Geometry: final body of the model. Coordinates: model frame, mm. A direction names the side the tool comes from. Give positions to 0.01 mm unless a question says otherwise; leave off trailing zeros. Order: outer loops, then holes, each group sorted by start corner. A loop starts at its lowest first (then second) coordinate and runs counter-clockwise, first axis right, second up. Notation, with made-up numbers: (60.5, 69) - (103.5, 69) arc R21 ccw to (103.5, 90) - close; hole circle Ø11 at (12.25, -26). An arc over 180 degrees is marked (long way). Use one line per item in the form item = value.
from build123d import *

# Parameters (mm, degrees)
F0_W      = 32
F0_H      = 9
F0_W_2    = 1
F1_DEPTH  = 6.5
F2_DEPTH  = 5.5
F3_DEPTH  = 4
F4_W      = 1
F4_H      = 1
F5_DEPTH  = 35
F6_DEPTH  = 33
F9_DEPTH  = 2
F4_W_2    = 9
F10_DEPTH = 33


with BuildPart() as f1:
    # F0 (on Top) → F1 (new body)
    with BuildSketch(Plane.XY):
        Polygon((4.2322745472, -4.5), (-27.7677254528, -4.5), (-28.7677254528, -4.5), (-28.7677254528, -6.5), (7.2322745472, -6.5), (7.2322745472, 6.5), (-28.7677254528, 6.5), (-28.7677254528, 4.5), (-27.7677254528, 4.5), (4.2322745472, 4.5), align=None)
        with Locations((-11.7677254528, 0)):
            Rectangle(F0_W, F0_H)
        with Locations((-28.2677254528, 0)):
            Rectangle(F0_W_2, F0_H)
    extrude(amount=F1_DEPTH)

    # F0 (on Top) → F2 (cut)
    with BuildSketch(Plane.XY):
        with Locations((-11.7677254528, 0)):
            Rectangle(F0_W, F0_H)
    extrude(amount=F2_DEPTH, mode=Mode.SUBTRACT)

    # F0 (on Top) → F3 (join)
    with BuildSketch(Plane.XY):
        Polygon((4.2322745472, -4.5), (-27.7677254528, -4.5), (-28.7677254528, -4.5), (-28.7677254528, -6.5), (7.2322745472, -6.5), (7.2322745472, 6.5), (-28.7677254528, 6.5), (-28.7677254528, 4.5), (-27.7677254528, 4.5), (4.2322745472, 4.5), align=None)
    extrude(amount=-F3_DEPTH)

    # F4 (on face) → F5 (cut)
    with BuildSketch(Plane(origin=(-28.7677254528, 0, 0), x_dir=(0, -1, 0), z_dir=(-1, 0, 0))):
        with Locations((-5, -1.5)):
            Rectangle(F4_W, F4_H)
    extrude(amount=-F5_DEPTH, mode=Mode.SUBTRACT)

    # F4 (on face) → F6 (cut)
    with BuildSketch(Plane(origin=(-28.7677254528, 0, 0), x_dir=(0, -1, 0), z_dir=(-1, 0, 0))):
        with Locations((-5, 1.5)):
            Rectangle(F4_W, F4_H)
        Polygon((-4.5, 1), (-4.5, 0), (0, 0), (0, 2), (-4.5, 2), align=None)
    extrude(amount=-F6_DEPTH, mode=Mode.SUBTRACT)

    # F7: F1 across plane


with BuildPart() as f1_1:
    add(f1.part)
    add(f1.part.mirror(Plane.XZ), mode=Mode.INTERSECT)

    # F8 (on face) → F9 (cut)
    with BuildSketch(Plane(origin=(4.2322745472, 0, 0), x_dir=(0, -1, 0), z_dir=(-1, 0, 0))):
        Polygon((4.5, 0), (-4.5, 0), (-4.5, -1), (-4.5, -2), (-4.5, -3), (4.5, -3), (4.5, -2), (4.5, -1), align=None)
    extrude(amount=-F9_DEPTH, mode=Mode.SUBTRACT)

    # F4 (on face) → F10 (join, through all)
    with BuildSketch(Plane(origin=(-28.7677254528, 0, 0), x_dir=(0, -1, 0), z_dir=(-1, 0, 0))):
        with Locations((0, -3.5)):
            Rectangle(F4_W_2, F4_H)
    extrude(amount=-F10_DEPTH)


solid = f1_1.part
(1) Pull-direction query (Z, two-part tool) for faces 3 (the face through (-28.768, 0.1, 2.5)), 4 (the face through (-14, 5, 2)), 5 (the face through (-11, 0, -4)); classes: released by +Z, released by -Z, zero draft, split by the parting line, or undercut.
Computed values:
face_3 = zero draft
face_4 = undercut
face_5 = released by -Z
(2) Cut plane D-D on z = -0.5. Output: boundary loops of the cut face in (x, y), plus the area to 3 significant figures.
Computed values:
outline = (-28.77, -6.5) - (7.23, -6.5) - (7.23, 6.5) - (-28.77, 6.5) - (-28.77, 4.5) - (6.23, 4.5) - (6.23, -4.5) - (-28.77, -4.5) - close
area = 153 mm²
(3) Cut plane B-B on x = -23.5. Output: boundary loops of the cut face in (y, z), plus the area to 3 significant figures.
Computed values:
outline = (-6.5, -4) - (6.5, -4) - (6.5, 6.5) - (-6.5, 6.5) - close; hole (-5.5, -2) - (-4.5, -2) - (-4.5, -3) - (4.5, -3) - (4.5, -2) - (5.5, -2) - (5.5, -1) - (4.5, -1) - (4.5, 1) - (5.5, 1) - (5.5, 2) - (4.5, 2) - (4.5, 5.5) - (-4.5, 5.5) - (-4.5, 2) - (-5.5, 2) - (-5.5, 1) - (-4.5, 1) - (-4.5, -1) - (-5.5, -1) - close
area = 56.0 mm²
(4) Cut plane A-A on z = 4. Output: boundary loops of the cut face in (x, y), plus the area to 3 significant figures.
Computed values:
outline = (-28.77, -6.5) - (7.23, -6.5) - (7.23, 6.5) - (-28.77, 6.5) - close; hole (-27.77, -4.5) - (4.23, -4.5) - (4.23, 4.5) - (-27.77, 4.5) - close
area = 180 mm²
(5) Ray query, line 1 along Z through (x, y) = (-19.5, 5); line 2 along Y through (x, z) = (0.5, 0.75); line 3 along Z through (x, y) = (-1.5, 1.75). Return the intervals inside material, ascending.
Computed values:
line_1 = -4 to -2, -1 to 1, 2 to 6.5
line_2 = -6.5 to -4.5, 4.5 to 6.5
line_3 = -4 to -3, 5.5 to 6.5
(6) Cut plane C-C on y = -0.25. Output: boundary loops of the cut face in (x, z), plus the area to 3 significant figures.
Computed values:
outline = (-28.77, -4) - (7.23, -4) - (7.23, 6.5) - (-28.77, 6.5) - (-28.77, 2) - (-27.77, 2) - (-27.77, 5.5) - (4.23, 5.5) - (4.23, 0) - (6.23, 0) - (6.23, -3) - (-28.77, -3) - close
area = 95.0 mm²
(7) Reachability of faces 1 (the face through (-12, 0, 5.5)), 2 (the face through (-11.5, 4.5, -2.5)) from +Z, -Z, +X, -X, +Y, -Y: full face, straight path, thin tool, end or side. Return the list, or none.
Computed values:
face_1 = none
face_2 = -X
